Read the model definition and answer for the solid it produces. Units are mm, in the model's axes. A direction names the side the tool comes from. Round coordinates to 2 decimals unless told otherwise and drop trailing zeros. Order: outer loops, then holes, each group sorted by start corner. A loop starts at its lowest first (then second) coordinate and runs counter-clockwise, first axis right, second up. Notation, with made-up numbers: (-34, 64.5) - (25, 64.5) arc R29 cw to (25, 103.5) - close; hole circle Ø9 at (74.25, 86.5). An arc over 180 degrees is marked (long way). One line per question, with ' | ' between items. Start each with the question number.
1) The mould has two halves that part along Y. Classify faces 1 (the cylindrical face through (-287.342, 25.609, 1.565)), 2 (the flat face through (-304.8, 2, 11)), 3 (the flat face through (4, 0, 19)), 4 (the flat face through (4, 3.175, 20)): pulls with the +Y half, pulls with the -Y half, needs draft (parallel to the pull), parting line crosses it, or undercut.
2) The part is cut by section A-A, the plane y = 14. Give the vertices of the cut face in (x, z) (3 decimals), plus the area to 3 significant figures.
3) For faces 5 (the flat face through (304.8, 2, 11)), 6 (the flat face through (4, 21, 3.175)), determine the directions among +Z, -Z, +X, -X, +Y, -Y from which every point of the face is accessible in a straight line to the end or side of a thin tool.
4) The part is cut by section B-B, the plane x = 43.5. Give the vertices of the cut face in (y, z) (3 decimals).
5) Straight lines are drawn through the part: line 1 (Y direction, x = -292.1, z = 2.45); line 2 (Z direction, x = -111, y = 8.5) (3 decimals). For each, find the intervals that lie inside material, in ascending order. Write a range as from..to.
6) Flat-ended cylindrical pins translate along their axes: pin 1 (6 mm diameter, centred on x = 13, z = 20.5, fed in from -Y); pin 2 (17.5 mm diameter, centred on x = 79.5, z = 13, fed in from +Y) (3 decimals). Find the tip coordinate at first contact, or state that the pin passes through.
from build123d import *

# Parameters (mm, degrees)
EXTRUDE_THIN1_DEPTH = 304.8
CUT_EXTRUDE1_REACH  = 311.526
SKETCH2_R           = 4.7625


with BuildPart() as part:
    # Sketch1 → Extrude-Thin1 (new, symmetric)
    with BuildSketch(Plane(origin=(0, 0, 0), x_dir=(0, 0, -1), z_dir=(1, 0, 0))):
        Polygon((-38.1, 0), (0, 0), (0, 38.1), (-3.175, 38.1), (-3.175, 3.175), (-38.1, 3.175), align=None)
    extrude(amount=EXTRUDE_THIN1_DEPTH, both=True)

    # Sketch2 → Cut-Extrude1 (cut, up to next)
    with BuildSketch(Plane(origin=(0, 0, 0), x_dir=(-1, 0, 0), z_dir=(0, 0, -1)), mode=Mode.PRIVATE) as cut_extrude1_sk1:
        with Locations((292.1, 25.4)):
            Circle(SKETCH2_R)
    cut_extrude1_tool1 = extrude(cut_extrude1_sk1.sketch, amount=-CUT_EXTRUDE1_REACH, mode=Mode.PRIVATE) & part.part
    add(cut_extrude1_tool1.solids().sort_by_distance((-292.1, 25.4, 0))[0], mode=Mode.SUBTRACT)


solid = part.part
Values:
1) face 1: undercut | face 2: needs draft | face 3: pulls with the -Y half | face 4: pulls with the +Y half
2) outline: (-304.8, 0) - (304.8, 0) - (304.8, 3.175) - (-304.8, 3.175) - close | area: 1,940 mm^2
3) face 5: +Z, -Z, +X, +Y, -Y | face 6: +Z, +X, -X, +Y
4) outline: (0, 0) - (38.1, 0) - (38.1, 3.175) - (3.175, 3.175) - (3.175, 38.1) - (0, 38.1) - close
5) line 1: y = 0..20.64, 30.16..38.1 | line 2: z = 0..3.175
6) pin 1: stops at y = 0 | pin 2: stops at y = 3.175
